```python
from build123d import *

# Parameters (mm, degrees)
BOSS_EXTRUDE1_DEPTH      = 5
BOSS_EXTRUDE1_DEPTH_BACK = 100
SKETCH1_R                = 14
SKETCH2_W                = 8
SKETCH2_H                = 24
CUT_EXTRUDE1_DEPTH       = 8
SKETCH3_R                = 14
BOSS_EXTRUDE2_DEPTH      = 8
FILLET1_R                = 4
SKETCH4_W                = 4
SKETCH4_H                = 3
SKETCH7_W                = 6.85
SKETCH7_H                = 2.4
CUT_EXTRUDE2_START       = -5
SKETCH8_R                = 14
CUT_EXTRUDE2_DEPTH       = 5
SKETCH9_R                = 21.936925755
SKETCH9_R_2              = 9.25
CUT_EXTRUDE3_DEPTH       = 28
BOSS_EXTRUDE3_START      = 30
SKETCH10_R               = 9.25
BOSS_EXTRUDE3_DEPTH      = 30
CHAMFER1_SIZE            = 1
CUT_EXTRUDE4_START       = 5
CUT_EXTRUDE4_DEPTH       = 10


with BuildPart() as part:
    # Sketch1 → Boss-Extrude1 (new, two sides: drawn at the far end of the back side and taken through both)
    with BuildSketch(Plane.XY.offset(-BOSS_EXTRUDE1_DEPTH_BACK)):
        Circle(SKETCH1_R)
    extrude(amount=BOSS_EXTRUDE1_DEPTH + BOSS_EXTRUDE1_DEPTH_BACK)

    # Sketch2 → Cut-Extrude1 (cut)
    with BuildSketch(Plane.XZ.offset(-17.3)):
        with Locations((0, -13.5)):
            Rectangle(SKETCH2_W, SKETCH2_H)
    extrude(amount=CUT_EXTRUDE1_DEPTH, mode=Mode.SUBTRACT)

    # Sketch3 → Boss-Extrude2 (add)
    with BuildSketch(Plane.XY.offset(5)):
        Circle(SKETCH3_R)
    extrude(amount=BOSS_EXTRUDE2_DEPTH)

    # Fillet1
    fillet1_edges = [part.edges().sort_by_distance(p)[0] for p in [
        (-4, 11.358203932, -25.5),
        (4, 11.358203932, -25.5),
        (4, 11.358203932, -1.5),
        (-4, 11.358203932, -1.5),
    ]]
    fillet(fillet1_edges, radius=FILLET1_R - 0.0001)  # a hair under: the kernel refuses the full size

    # Sketch4 → Revolve1 (revolve)
    with BuildSketch(Plane(origin=(0, 0, 0), x_dir=(0, 0, -1), z_dir=(1, 0, 0)), mode=Mode.PRIVATE) as revolve1_sk:
        with Locations((-2, -15.5)):
            Rectangle(SKETCH4_W, SKETCH4_H)
    revolve(revolve1_sk.sketch.rotate(Axis((0, 0, 0), (0, 0, -1)), 270), axis=Axis((0, 0, 0), (0, 0, -1)))

    # Sketch7 → Cut-Revolve2 (revolve, cut)
    with BuildSketch(Plane(origin=(0, 0, 0), x_dir=(1, 0, 0), z_dir=(0, 1, 0)), mode=Mode.PRIVATE) as cut_revolve2_sk:
        with Locations((-16.575, 28.197290459)):
            Rectangle(SKETCH7_W, SKETCH7_H)
    revolve(cut_revolve2_sk.sketch.rotate(Axis((0, 0, 5), (0, 0, -1)), 180), axis=Axis((0, 0, 5), (0, 0, -1)), mode=Mode.SUBTRACT)

    # Sketch8 → Cut-Extrude2 (cut)
    with BuildSketch(Plane.XY.offset(13).offset(CUT_EXTRUDE2_START)):
        Circle(SKETCH8_R)
    extrude(amount=CUT_EXTRUDE2_DEPTH, mode=Mode.SUBTRACT)

    # Sketch9 → Cut-Extrude3 (cut)
    with BuildSketch(Plane(origin=(0, 0, -100), x_dir=(-1, 0, 0), z_dir=(0, 0, -1))):
        Circle(SKETCH9_R)
        Circle(SKETCH9_R_2, mode=Mode.SUBTRACT)
    extrude(amount=-CUT_EXTRUDE3_DEPTH, mode=Mode.SUBTRACT)

    # Sketch10 → Boss-Extrude3 (add)
    with BuildSketch(Plane(origin=(0, 0, -100), x_dir=(-1, 0, 0), z_dir=(0, 0, -1)).offset(BOSS_EXTRUDE3_START)):
        Circle(SKETCH10_R)
    extrude(amount=-BOSS_EXTRUDE3_DEPTH)

    # Chamfer1
    chamfer1_edges = [part.edges().sort_by_distance(p)[0] for p in [
        (9.25, 0, -130),
        (-14, 0, 8),
    ]]
    chamfer(chamfer1_edges, length=CHAMFER1_SIZE)

    # Sketch15 → Cut-Extrude4 (cut)
    with BuildSketch(Plane(origin=(0, 0, 0), x_dir=(1, 0, 0), z_dir=(0, 1, 0)).offset(CUT_EXTRUDE4_START)):
        with BuildLine():
            Line((3, 122), (3, 102))
            ThreePointArc((3, 102), (0, 99), (-3, 102))
            Line((-3, 102), (-3, 122))
            ThreePointArc((-3, 122), (0, 125), (3, 122))
        make_face()
    extrude(amount=CUT_EXTRUDE4_DEPTH, mode=Mode.SUBTRACT)


solid = part.part
```
Model file for the job. Use its own axes, mm. A direction names the side the tool comes from. Round coordinates to 2 decimals unless told otherwise and drop trailing zeros. Order: outer loops, then holes, each group sorted by start corner. A loop starts at its lowest first (then second) coordinate and runs counter-clockwise, first axis right, second up. Notation, with made-up numbers: M 66.25,62.5 L 90.25,62.5 A28 ccw 90.25,90.5 Z; hole C 49.5,26.25 d1. An arc over 180 degrees is marked long. Use CSV: the item, a comma, the result in double quotes.
Item 1: Which spindle directions (+Z, -Z, +X, -X, +Y, -Y) get a long thin tool onto all of the face, cutting with end or side? Do faces 4 (the face through (6.5, -12.4, -13.7)), 5 (the face through (4, -13, -26.997)), 6 (the face through (-4, 11, -14)). Say none if no direction does.
Worked answers:
face 4,"-Z"
face 5,"none"
face 6,"+Y"
Item 2: Probe probe 1 along Z at (x, y) = (12, -1.5); probe 2 along Z at (x, y) = (-12, 10.5); probe 3 along X at (y, z) = (0, -26). List the from-to ranges inside material, lowest first.
Worked answers:
probe 1,"-72 to 8"
probe 2,"0 to 4"
probe 3,"-14 to 14"
Item 3: Saw through at B-B (z = -19.5). List the corners of the cut face in (x, y), plus the area to 3 significant figures.
Worked answers:
outline,"M -4,9.3 L -4,13.42 A14 ccw long 4,13.42 L 4,9.3 Z"
area,"580 mm²"
Item 4: Pull direction Z, two halves, no side cores. Call faces 1 (the face through (0, 0, 8)), 2 (the face through (2.797, 11.617, -2.641)), 3 (the face through (-3, -9, -72)): released by +Z, released by -Z, zero draft, split by the parting line, or undercut.
Worked answers:
face 1,"released by +Z"
face 2,"undercut"
face 3,"released by -Z"
Item 5: Saw through at A-A (z = -94). List the corners of the cut face in (x, y).
Worked answers:
outline,"C 0,0 d18.5"
Item 6: Saw through at D-D (z = -118.5). List the corners of the cut face in (x, y).
Worked answers:
outline,"M -3,5 L -3,8.75 A9.25 ccw long 3,8.75 L 3,5 Z"
Item 7: Pin check, flat tips, straight feed: pin 1 (2 mm diameter, centred on y = 11, z = -12.5, fed in from -X); pin 2 (4 mm diameter, centred on y = 6.5, z = -116.5, fed in from -X); pin 3 (1 mm diameter, centred on x = -9.5, y = 10, fed in from +Z). Stop position of each tip, or through.
Worked answers:
pin 1,"x = -9.8"
pin 2,"x = -8.08"
pin 3,"z = 7.71"
Item 8: Saw through at C-C (z = -50). List the corners of the cut face in (x, y).
Worked answers:
outline,"C 0,0 d28"
